```python
from build123d import *

# Parameters (mm, degrees)
SKETCH_2_W                = 9.215
SKETCH_2_H                = 29.4
EXTRUDE_1_DEPTH           = 3.7
SKETCH_2_5_W              = 8.42
SKETCH_2_5_H              = 28.6
CUT_EXTRUDE_2_DEPTH       = 3.3
CUT_EXTRUDE_7_DEPTH       = 32.031697102
CUT_EXTRUDE_7_DEPTH_BACK  = 0.4
SKETCH_3_W                = 6.915
SKETCH_3_H                = 1.1
CUT_EXTRUDE_11_DEPTH      = 32.031697102
CUT_EXTRUDE_11_DEPTH_BACK = 0.4
SKETCH_14_W               = 7.7
SKETCH_14_H               = 1.1
SKETCH_14_W_2             = 7.5
SKETCH_14_W_3             = 9.1
CUT_EXTRUDE_12_DEPTH      = 10


with BuildPart() as part:
    # 草图2 → 凸台-拉伸1 (new body)
    with BuildSketch(Plane(origin=(0, 0, 0), x_dir=(1, 0, 0), z_dir=(0, 1, 0))):
        with Locations((4.6075, 14.7)):
            Rectangle(SKETCH_2_W, SKETCH_2_H)
    extrude(amount=EXTRUDE_1_DEPTH)

    # 草图2<5> → 切除-拉伸2 (cut)
    with BuildSketch(Plane(origin=(0, 0, 0), x_dir=(1, 0, 0), z_dir=(0, 1, 0))):
        with Locations((4.61, 14.7)):
            Rectangle(SKETCH_2_5_W, SKETCH_2_5_H)
    extrude(amount=CUT_EXTRUDE_2_DEPTH, mode=Mode.SUBTRACT)

    # 草图3 → 切除-拉伸7 (cut, two sides: drawn at the far end of the back side and taken through both)
    with BuildSketch(Plane.XY.offset(-CUT_EXTRUDE_7_DEPTH_BACK)):
        with Locations((4.6075, 0.55)):
            Rectangle(SKETCH_3_W, SKETCH_3_H)
    extrude(amount=CUT_EXTRUDE_7_DEPTH + CUT_EXTRUDE_7_DEPTH_BACK, mode=Mode.SUBTRACT)

    # 草图8 → 切除-拉伸11 (cut, two sides: drawn at the far end of the back side and taken through both)
    with BuildSketch(Plane(origin=(0, 0, -29.4), x_dir=(-1, 0, 0), z_dir=(0, 0, -1)).offset(-CUT_EXTRUDE_11_DEPTH_BACK)):
        Polygon((-39.075133434, 0), (-9.215, 0), (-8.065, 0), (-8.065, 1.1), (-1.15, 1.1), (-1.15, 0), (0, 0), (29.860133434, 0), (29.860133434, -59.720266867), (-39.075133434, -59.720266867), align=None)
    extrude(amount=CUT_EXTRUDE_11_DEPTH + CUT_EXTRUDE_11_DEPTH_BACK, mode=Mode.SUBTRACT)

    # 草图14 → 切除-拉伸12 (cut)
    with BuildSketch(Plane.ZY):
        with Locations((-24.4, 0.55)):
            Rectangle(SKETCH_14_W, SKETCH_14_H)
        with Locations((-15.4, 0.55)):
            Rectangle(SKETCH_14_W_2, SKETCH_14_H)
        with Locations((-5.7, 0.55)):
            Rectangle(SKETCH_14_W_3, SKETCH_14_H)
    extrude(amount=-CUT_EXTRUDE_12_DEPTH, mode=Mode.SUBTRACT)


solid = part.part
```
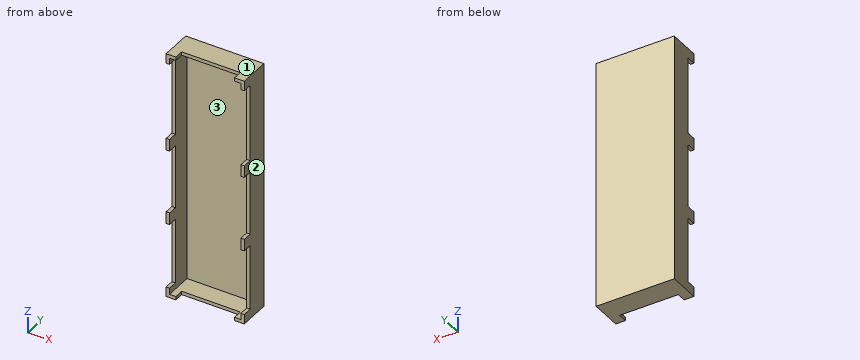
Could you check a few things on this model? Use its own coordinates, in mm. Face numbers are marked on the shaded views. Round coordinates to 2 decimals unless told otherwise and drop trailing zeros. Write each loop counter-clockwise with the first axis right and the second up, starting at its lowest first coordinate (ties: lowest second). Pieces come first, ordered by that corner, then holes. Notation, with made-up numbers: M 78.25,7 L 126.25,7 A23 cw 126.25,19 Z; hole C 6.25,81 d4. An arc over 180 degrees is marked long. Answer in a Markdown table with one row per item. Add a question column.
Q1. If we mould it in two halves opening along X, with no side actions, what happens to the marked faces 1, 2 and 3? For each: +X half, -X half, draft (parallel to the pull), parting line (faces both ways), or undercut.
Q2. Imagine slicing it at C-C (z = -7.75). Please give me the cut outline in (x, y) (3 decimals).
Q3. Imagine slicing it at B-B (y = 1.6). Please give me the cut outline in (x, z) (3 decimals).
Q4. Imagine slicing it at A-A (x = 5). Please give me the cut outline in (y, z).
Q5. Will this pin go through, and if not, where does the flat tip stop? pin 1 Ø4 at (x, z) = (4.5, -20.5) entering from -Y.
Q6. If I drill on line 1 (X direction, y = 1.3, z = -13.75) (3 decimals); line 2 (Z direction, x = 0.5, y = 0.9); line 3 (Y direction, x = 4.75, z = -12.75), over which ranges is the centre line in solid material (lowest first)? Write a range as from..to.
Values:
| question | item | result |
|---|---|---|
| 1 | face 1 | draft |
| 1 | face 2 | +X half |
| 1 | face 3 | undercut |
| 2 | outline | M 0,1.1 L 0.4,1.1 L 0.4,3.3 L 8.82,3.3 L 8.82,1.1 L 9.215,1.1 L 9.215,3.7 L 0,3.7 Z |
| 3 | outline | M 0,-29.4 L 9.215,-29.4 L 9.215,0 L 0,0 Z; hole M 0.4,-29 L 8.82,-29 L 8.82,-0.4 L 0.4,-0.4 Z |
| 4 | outline | M 1.1,-29.4 L 3.7,-29.4 L 3.7,0 L 1.1,0 L 1.1,-0.4 L 3.3,-0.4 L 3.3,-29 L 1.1,-29 Z |
| 5 | pin 1 | y = 3.3 |
| 6 | line 1 | 0..0.4, 8.82..9.215 |
| 6 | line 2 | -29.4..-29, -0.4..0 |
| 6 | line 3 | 3.3..3.7 |
